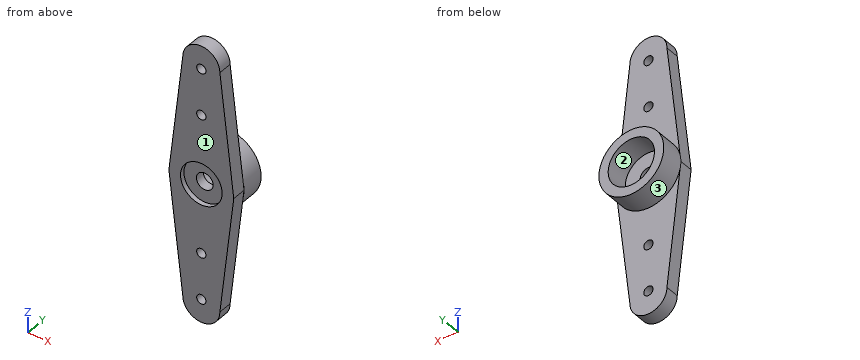
from build123d import *

# Parameters (mm, degrees)
EXTRUDE_2_DEPTH     = 1.5
SKETCH_7_R          = 3.5
EXTRUDE_3_DEPTH     = 2.5
SKETCH_8_R          = 2.5
CUT_EXTRUDE_1_DEPTH = 2.5
SKETCH_9_R          = 2.25
CUT_EXTRUDE_2_DEPTH = 0.5
SKETCH_10_R         = 0.9
CUT_EXTRUDE_3_DEPTH = 1
SKETCH_11_R         = 0.5
CUT_EXTRUDE_4_DEPTH = 1.5


with BuildPart() as part:
    # Эскиз1 → Бобышка-Вытянуть2 (new body)
    with BuildSketch(Plane(origin=(0, 0, 0), x_dir=(1, 0, 0), z_dir=(0, 1, 0))):
        with BuildLine():
            ThreePointArc((2, 13), (0, 15), (-2, 13))
            Line((-2, 13), (-3.5, 0))
            Line((-3.5, 0), (-2, -13))
            ThreePointArc((-2, -13), (0, -15), (2, -13))
            Line((2, -13), (3.5, 0))
            Line((3.5, 0), (2, 13))
        make_face()
    extrude(amount=EXTRUDE_2_DEPTH)

    # Эскиз7 → Бобышка-Вытянуть3 (add)
    with BuildSketch(Plane(origin=(0, 1.5, 0), x_dir=(1, 0, 0), z_dir=(0, 1, 0))):
        Circle(SKETCH_7_R)
    extrude(amount=EXTRUDE_3_DEPTH)

    # Эскиз8 → Вырез-Вытянуть1 (cut)
    with BuildSketch(Plane(origin=(0, 4, 0), x_dir=(1, 0, 0), z_dir=(0, 1, 0))):
        Circle(SKETCH_8_R)
    extrude(amount=-CUT_EXTRUDE_1_DEPTH, mode=Mode.SUBTRACT)

    # Эскиз9 → Вырез-Вытянуть2 (cut)
    with BuildSketch(Plane.XZ):
        Circle(SKETCH_9_R)
    extrude(amount=-CUT_EXTRUDE_2_DEPTH, mode=Mode.SUBTRACT)

    # Эскиз10 → Вырез-Вытянуть3 (cut)
    with BuildSketch(Plane.XZ.offset(-0.5)):
        Circle(SKETCH_10_R)
    extrude(amount=-CUT_EXTRUDE_3_DEPTH, mode=Mode.SUBTRACT)

    # Эскиз11 → Вырез-Вытянуть4 (cut)
    with BuildSketch(Plane.XZ):
        with Locations((0, -7.5)):
            Circle(SKETCH_11_R)
        with Locations((0, -12.5)):
            Circle(SKETCH_11_R)
        with Locations((0, 12.5)):
            Circle(SKETCH_11_R)
        with Locations((0, 7.5)):
            Circle(SKETCH_11_R)
    extrude(amount=-CUT_EXTRUDE_4_DEPTH, mode=Mode.SUBTRACT)


solid = part.part
Geometry check sheet. Reference: the model listing, model coordinates, mm. Face numbers are marked on the shaded views. Coordinates: 2 decimals unless noted, no trailing zeros. Write each loop counter-clockwise with the first axis right and the second up, starting at its lowest first coordinate (ties: lowest second). Pieces come first, ordered by that corner, then holes. Notation, with made-up numbers: (1.5, 35) -> (33.5, 35) arc R10 ccw to (33.5, 41) -> close; hole circle Ø10 at (-15.5, 28.25). An arc over 180 degrees is marked (long way). One line per question, with ' | ' between items.
1. Cross-section at C-C on y = 2.3. Record the cut outline in (x, z), and give its area (3 significant figures).
Answers:
outline: circle Ø7 at (0, 0); hole circle Ø5 at (0, 0) | area: 18.8 mm²
2. Cross-section at A-A on z = 12.5. Record the cut outline in (x, y), and give its area (3 significant figures).
Answers:
outline: (-2.06, 0) -> (-0.5, 0) -> (-0.5, 1.5) -> (-2.06, 1.5) -> close; (0.5, 0) -> (2.06, 0) -> (2.06, 1.5) -> (0.5, 1.5) -> close | area: 4.67 mm²
3. Draft check along X on the marked faces 1, 2 and 3. Enter one of: +X half, -X half, draft (parallel to the pull), parting line (faces both ways), or undercut.
Answers:
face 1: draft | face 2: undercut | face 3: parting line
4. Thickness scan on probe 1 along Z at (x, y) = (0, 1); probe 2 along Z at (x, y) = (0, 0.35); probe 3 along Z at (x, y) = (0, 3.45). Record the ranges inside material, lowest first. Write a range as from..to.
Answers:
probe 1: z = -15..-13, -12..-8, -7..-0.9, 0.9..7, 8..12, 13..15 | probe 2: z = -15..-13, -12..-8, -7..-2.25, 2.25..7, 8..12, 13..15 | probe 3: z = -3.5..-2.5, 2.5..3.5
5. Depth check by flat-ended pin: pin 1 Ø4 at (x, z) = (0, 0) entering from +Y; pin 2 Ø1.3 at (x, z) = (-0.5, -0.5) entering from -Y; pin 3 Ø2 at (x, y) = (2, 3.5) entering from +Z. Enter the tip coordinate at first touch or a pass-through.
Answers:
pin 1: stops at y = 1.5 | pin 2: stops at y = 0.5 | pin 3: stops at z = 3.35
6. Cross-section at B-B on x = 0. State how many separate pieces and enclosed holes the cut face has, and give its area (4 significant figures).
Answers:
separate pieces: 6 | enclosed holes: 0 | area: 39.95 mm²
